```python
from build123d import *

# Parameters (mm, degrees)
SKETCH1_W           = 250
SKETCH1_H           = 250
BOSS_EXTRUDE1_DEPTH = 50
BOSS_EXTRUDE2_DEPTH = 25
SKETCH8_R           = 5
CUT_EXTRUDE1_DEPTH  = 25
SKETCH9_W           = 242
SKETCH9_H           = 242
CUT_EXTRUDE4_DEPTH  = 46
EXTRUDE_THIN2_DEPTH = 46
SKETCH15_R          = 11
CUT_EXTRUDE5_DEPTH  = 4
SKETCH17_W          = 15
SKETCH17_H          = 55
CUT_EXTRUDE7_DEPTH  = 4
SKETCH18_W          = 10
SKETCH18_H          = 16.5
CUT_EXTRUDE8_DEPTH  = 2.5
FILLET1_R           = 10
FILLET2_R           = 10


with BuildPart() as part:
    # Sketch1 → Boss-Extrude1 (new body)
    with BuildSketch(Plane.XY):
        with Locations((125, 125)):
            Rectangle(SKETCH1_W, SKETCH1_H)
    extrude(amount=BOSS_EXTRUDE1_DEPTH)

    # Sketch5 → Boss-Extrude2 (add)
    with BuildSketch(Plane.XY):
        with BuildLine():
            Line((105, 250), (105, 265))
            ThreePointArc((105, 265), (105.585786438, 266.414213562), (107, 267))
            Line((107, 267), (143, 267))
            ThreePointArc((143, 267), (144.414213562, 266.414213562), (145, 265))
            Line((145, 265), (145, 250))
            Line((145, 250), (105, 250))
        make_face()
    boss_extrude2 = extrude(amount=BOSS_EXTRUDE2_DEPTH)

    # Mirror1: Boss-Extrude2 across plane
    add(boss_extrude2.mirror(Plane.ZX.offset(125)))

    # Sketch8 → Cut-Extrude1 (cut)
    with BuildSketch(Plane(origin=(0, 0, 0), x_dir=(-1, 0, 0), z_dir=(0, 0, -1))):
        with Locations((-125, -7.5)):
            Circle(SKETCH8_R)
        with Locations((-125, 257.5)):
            Circle(SKETCH8_R)
    extrude(amount=-CUT_EXTRUDE1_DEPTH, mode=Mode.SUBTRACT)

    # Sketch9 → Cut-Extrude4 (cut)
    with BuildSketch(Plane(origin=(0, 0, 0), x_dir=(-1, 0, 0), z_dir=(0, 0, -1))):
        with Locations((-125, 125)):
            Rectangle(SKETCH9_W, SKETCH9_H)
    extrude(amount=-CUT_EXTRUDE4_DEPTH, mode=Mode.SUBTRACT)

    # Sketch14 → Extrude-Thin2 (add)
    with BuildSketch(Plane(origin=(0, 0, 0), x_dir=(-1, 0, 0), z_dir=(0, 0, -1))):
        Polygon((-4, 49), (-54, 49), (-54, 4), (-56.5, 4), (-56.5, 51.5), (-4, 51.5), align=None)
    extrude(amount=-EXTRUDE_THIN2_DEPTH)

    # Sketch15 → Cut-Extrude5 (cut)
    with BuildSketch(Plane.ZY):
        with Locations((26, 24)):
            Circle(SKETCH15_R)
    extrude(amount=-CUT_EXTRUDE5_DEPTH, mode=Mode.SUBTRACT)

    # Sketch17 → Cut-Extrude7 (cut)
    with BuildSketch(Plane(origin=(250, 0, 0), x_dir=(0, 0, -1), z_dir=(1, 0, 0))):
        with Locations((-18.5, 125)):
            Rectangle(SKETCH17_W, SKETCH17_H)
    extrude(amount=-CUT_EXTRUDE7_DEPTH, mode=Mode.SUBTRACT)

    # Sketch18 → Cut-Extrude8 (cut)
    with BuildSketch(Plane(origin=(0, 51.5, 0), x_dir=(1, 0, 0), z_dir=(0, 1, 0))):
        with Locations((40.5, -37.75)):
            Rectangle(SKETCH18_W, SKETCH18_H)
    extrude(amount=-CUT_EXTRUDE8_DEPTH, mode=Mode.SUBTRACT)

    # Fillet1
    fillet1_edges = [part.edges().sort_by_distance(p)[0] for p in [
        (0, 250, 25),
        (250, 250, 25),
        (250, 0, 25),
        (0, 0, 25),
    ]]
    fillet(fillet1_edges, radius=FILLET1_R)

    # Fillet2
    fillet2_edges = [part.edges().sort_by_distance(p)[0] for p in [
        (246, 246, 23),
        (4, 246, 23),
        (4, 4, 23),
        (246, 4, 23),
    ]]
    fillet(fillet2_edges, radius=FILLET2_R)


solid = part.part
```
Geometry check sheet. Reference: the model listing, model coordinates, mm. A direction names the side the tool comes from. Give positions to 0.01 mm unless a question says otherwise; leave off trailing zeros. Order: outer loops, then holes, each group sorted by start corner. A loop starts at its lowest first (then second) coordinate and runs counter-clockwise, first axis right, second up.
1. Gauge pin test, flat ends, axial feed: pin 1 Ø3 at (x, y) = (182, 67) entering from -Z; pin 2 Ø1.2 at (x, z) = (247, 20) entering from +Y; pin 3 Ø1.2 at (x, z) = (247, 21) entering from -Y. Record the tip position at first contact, or that the pin passes through.
2. Section check B-B, the plane x = 125. Enter the section's corners in (y, z), and give its area (3 significant figures).
3. Section check C-C, the plane x = 50. Enter the section's corners in (y, z).
4. Section check D-D, the plane y = 257.5. Enter the section's corners in (x, z).
5. Section check A-A, the plane y = 24. Enter the section's corners in (x, z), and give its area (4 significant figures).
6. Release check for a two-part mould opening along X. For faces 1 (the face through (123, 127, 50)), 2 (the face through (148, 4, 23)), 3 (the face through (105, -7, 12)) record: pulls with the +X half, pulls with the -X half, needs draft (parallel to the pull), parting line crosses it, or undercut.
7. Thickness scan on L1, parallel to Y at x = 125, z = 14; L2, parallel to X at y = 30.5, z = 11.5; L3, parallel to Y at x = 25, z = 45. Record the ranges inside material, lowest first.
8. Access from +Z, -Z, +X, -X, +Y, -Y to the whole of each face (thin tool, end or side, straight path). Record for faces 4 (the face through (145, 258, 12)), 5 (the face through (120.23, -6, 12.32)), 6 (the face through (243.15, 242.99, 23.32)).
Values follow:
1. pin 1: stops at z = 46
1. pin 2: stops at y = 247.68
1. pin 3: stops at y = 2.32
2. outline: (-17, 0) - (-12.5, 0) - (-12.5, 25) - (-17, 25) - close; (-2.5, 0) - (4, 0) - (4, 46) - (246, 46) - (246, 0) - (252.5, 0) - (252.5, 25) - (250, 25) - (250, 50) - (0, 50) - (0, 25) - (-2.5, 25) - close; (262.5, 0) - (267, 0) - (267, 25) - (262.5, 25) - close
2. area: 1,720 mm2
3. outline: (0, 0) - (4, 0) - (4, 46) - (49, 46) - (49, 0) - (51.5, 0) - (51.5, 46) - (246, 46) - (246, 0) - (250, 0) - (250, 50) - (0, 50) - close
4. outline: (105, 0) - (120, 0) - (120, 25) - (105, 25) - close; (130, 0) - (145, 0) - (145, 25) - (130, 25) - close
5. outline: (0, 0) - (4, 0) - (4, 15) - (0, 15) - close; (0, 37) - (4, 37) - (4, 46) - (54, 46) - (54, 0) - (56.5, 0) - (56.5, 46) - (246, 46) - (246, 0) - (250, 0) - (250, 50) - (0, 50) - close
5. area: 1,395 mm2
6. face 1: needs draft
6. face 2: undercut
6. face 3: pulls with the -X half
7. L1: y = -17 to -12.5, -2.5 to 4, 246 to 252.5, 262.5 to 267
7. L2: x = 0 to 4, 54 to 56.5, 246 to 250
7. L3: y = 0 to 4, 49 to 51.5, 246 to 250
8. face 4: +Z, -Z, +X, +Y
8. face 5: +Z, -Z
8. face 6: -Z
